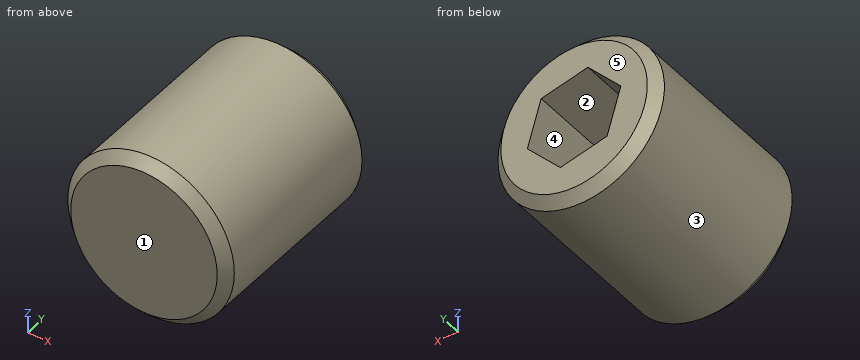
```python
from build123d import *

# Parameters (mm, degrees)
F0_R     = 2.5
F1_DEPTH = 6
F2_SIZE  = 0.3
F4_DEPTH = 3


with BuildPart() as f1:
    # F0 (on Front) → F1 (new body)
    with BuildSketch(Plane.XZ):
        Circle(F0_R)
    extrude(amount=F1_DEPTH)

    # F2
    f2_edges = [f1.edges().sort_by_distance(p)[0] for p in [
        (-2.5, -6, 0),
        (-2.5, 0, 0),
    ]]
    chamfer(f2_edges, length=F2_SIZE)

    # F3 (on face) → F4 (cut)
    with BuildSketch(Plane(origin=(0, 0, 0), x_dir=(-1, 0, 0), z_dir=(0, 1, 0))):
        Polygon((0.414277, 1.382645), (-0.990268, 1.050097), (-1.404544, -0.332549), (-0.414277, -1.382645), (0.990268, -1.050097), (1.404544, 0.332549), align=None)
    extrude(amount=-F4_DEPTH, mode=Mode.SUBTRACT)


solid = f1.part
```
CAD build for the part. Positions are in the model's coordinates, mm. Face numbers are marked on the shaded views. A direction names the side the tool comes from. Round coordinates to 2 decimals unless told otherwise and drop trailing zeros. Order: outer loops, then holes, each group sorted by start corner. A loop starts at its lowest first (then second) coordinate and runs counter-clockwise, first axis right, second up. Notation, with made-up numbers: (-32.75, 15) - (18.25, 15) arc R31 cw to (18.25, 53) - close; hole circle Ø9 at (27.25, 58). An arc over 180 degrees is marked (long way). Answer in a Markdown table with one row per item. Add a question column.
(1) Band-saw the part on A-A on y = -1.35. List the corners of the cut face in (x, z), and give its area (3 significant figures).
(2) Band-saw the part on C-C on x = 0. List the corners of the cut face in (y, z).
(3) Probe L1, parallel to X at y = -2.35, z = 0.65; L2, parallel to X at y = -1.1, z = -0.75; L3, parallel to Y at x = 0.9, z = 0.6. List the from-to ranges inside material, lowest first. Write a range as [from, to].
(4) Mould opens along Z. For the marked faces 1, 2 and 3 say: +Z half, -Z half, draft (parallel to the pull), parting line (faces both ways), or undercut.
(5) Drop flat-ended pins along their axis: pin 1 Ø1.5 at (x, y) = (-1, -5) entering from -Z; pin 2 Ø2 at (y, z) = (-1.5, -2) entering from -X. Give the stop position or say it passes through.
(6) 3-axis set-ups, long thin cutter, end or side, ignore diameter. For the marked faces 4 and 5: which of +Z, -Z, +X, -X, +Y, -Y reach the whole face in a straight line?
(7) Band-saw the part on D-D on y = -5.05. List the corners of the cut face in (x, z).
(8) Band-saw the part on B-B on z = 0. List the corners of the cut face in (x, y).
Data:
| question | item | result |
|---|---|---|
| 1 | outline | circle Ø5 at (0, 0); hole (-1.4, 0.33) - (-0.99, -1.05) - (0.41, -1.38) - (1.4, -0.33) - (0.99, 1.05) - (-0.41, 1.38) - close |
| 1 | area | 14.2 mm^2 |
| 2 | outline | (-6, -2.2) - (-5.7, -2.5) - (-0.3, -2.5) - (0, -2.2) - (0, -1.28) - (-3, -1.28) - (-3, 1.28) - (0, 1.28) - (0, 2.2) - (-0.3, 2.5) - (-5.7, 2.5) - (-6, 2.2) - close |
| 3 | L1 | x = [-2.41, -1.11], [1.11, 2.41] |
| 3 | L2 | x = [-2.38, -1.08], [1.01, 2.38] |
| 3 | L3 | y = [-6, -3] |
| 4 | face 1 | draft |
| 4 | face 2 | undercut |
| 4 | face 3 | parting line |
| 5 | pin 1 | stops at z = -2.49 |
| 5 | pin 2 | stops at x = -2.29 |
| 6 | face 4 | +Y |
| 6 | face 5 | +Z, -Z, +X, -X, +Y |
| 7 | outline | circle Ø5 at (0, 0) |
| 8 | outline | (-2.5, -5.7) - (-2.2, -6) - (2.2, -6) - (2.5, -5.7) - (2.5, -0.3) - (2.2, 0) - (1.3, 0) - (1.3, -3) - (-1.3, -3) - (-1.3, 0) - (-2.2, 0) - (-2.5, -0.3) - close |
